Can you work these out from the model? Positions are in its coordinate system, mm. Face numbers are marked on the shaded views. Give positions to 0.01 mm unless a question says otherwise; leave off trailing zeros. Write each loop counter-clockwise with the first axis right and the second up, starting at its lowest first coordinate (ties: lowest second). Pieces come first, ordered by that corner, then holes.
1. Suppose I cut it at A-A (z = 49). Please give me the cut outline in (x, y), and give its area (3 significant figures).
2. Thinking about a two-plate mould opening in X: for the marked faces 1, 2 and 3, which applies, pulls with the +X half, pulls with the -X half, needs draft (parallel to the pull), parting line crosses it, or undercut?
3. Suppose I cut it at C-C (y = -28.5). Please give me the cut outline in (x, z).
4. If I drill on probe 1 along Z at (x, y) = (35, 15); probe 2 along X at (y, z) = (30.5, 16); probe 3 along Z at (x, y) = (10, 5.5), over which ranges is the centre line in solid material (lowest first)?
5. Suppose I cut it at B-B (z = 8). Please give me the cut outline in (x, y), and give its area (3 significant figures).
6. I'm going to push flat-ended pins straight in: pin 1 (1.8 mm diameter, centred on x = 0, y = 38, fed in from +Z); pin 2 (10 mm diameter, centred on x = -18.5, z = 27.5, fed in from -Y); pin 3 (20 mm diameter, centred on x = -6, z = 13, fed in from +Y). Where does each tip first touch, or does it pass through?
7. Suppose I cut it at D-D (x = 10). Please give me the cut outline in (y, z), and give its area (3 significant figures).
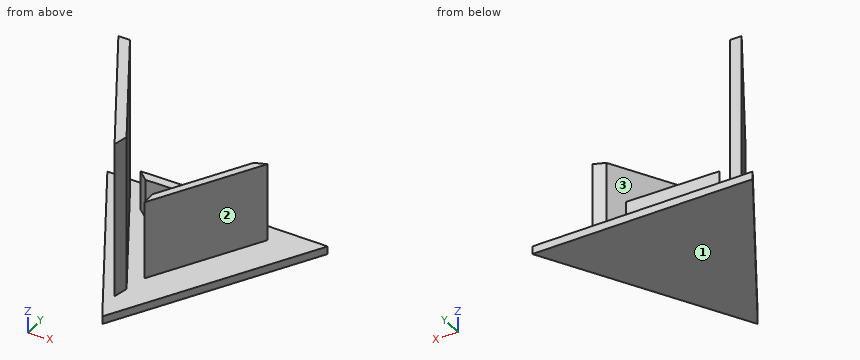
```python
from build123d import *

# Parameters (mm, degrees)
F1_DEPTH = 5
F3_DEPTH = 100
F4_DEPTH = 50
F5_DEPTH = 25


with BuildPart() as f1:
    # F0 (on Top) → F1 (new body)
    with BuildSketch(Plane.XY):
        Polygon((-1.194454, -60.107594), (70.600725, 60.107594), (-69.406271, 62.176449), align=None)
    extrude(amount=F1_DEPTH)

    # F2 (on face) → F3 (join)
    with BuildSketch(Plane.XY.offset(5)):
        Polygon((-48.847037, 51.363251), (-56.216117, 51.472142), (-5.24076, -39.911917), (-3.140415, -30.575492), align=None)
    extrude(amount=F3_DEPTH)

    # F2 (on face) → F4 (join)
    with BuildSketch(Plane.XY.offset(5)):
        Polygon((0, -7.590361), (0, -16.841115), (39.198391, 48.793401), (32.101094, 46.160308), align=None)
    extrude(amount=F4_DEPTH)

    # F2 (on face) → F5 (join)
    with BuildSketch(Plane.XY.offset(5)):
        Polygon((23.482682, 39.849401), (-35.579819, 39.849401), (-28.938254, 33.985027), (19.980348, 33.985027), align=None)
    extrude(amount=F5_DEPTH)


solid = f1.part
```
Checks:
1. outline: (-56.22, 51.47) - (-5.24, -39.91) - (-3.14, -30.58) - (-48.85, 51.36) - close; (0, -16.84) - (39.2, 48.79) - (32.1, 46.16) - (0, -7.59) - close
1. area: 963 mm2
2. face 1: needs draft
2. face 2: pulls with the +X half
2. face 3: undercut
3. outline: (-18.83, 0) - (17.68, 0) - (17.68, 5) - (-4.3, 5) - (-4.3, 105) - (-11.61, 105) - (-11.61, 5) - (-18.83, 5) - close
4. probe 1: z = 0 to 5
4. probe 2: x = -44.52 to -37.21, 22.75 to 28.27
4. probe 3: z = 0 to 55
5. outline: (-56.22, 51.47) - (-5.24, -39.91) - (-3.14, -30.58) - (-48.85, 51.36) - close; (-35.58, 39.85) - (-28.94, 33.99) - (19.98, 33.99) - (23.48, 39.85) - close; (0, -16.84) - (39.2, 48.79) - (32.1, 46.16) - (0, -7.59) - close
5. area: 1,280 mm2
6. pin 1: stops at z = 30
6. pin 2: stops at y = -25.11
6. pin 3: stops at y = 61.33
7. outline: (-41.36, 0) - (61, 0) - (61, 5) - (39.85, 5) - (39.85, 30) - (33.99, 30) - (33.99, 5) - (9.15, 5) - (9.15, 55) - (-0.1, 55) - (-0.1, 5) - (-41.36, 5) - close
7. area: 1,120 mm2
